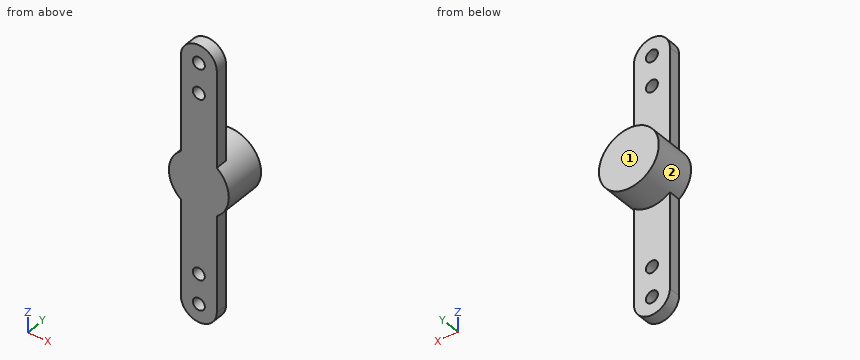
Autodesk Inventor part; units mm, degrees
ref_plane "YZ Plane" through (0, 0, 0) normal (1, 0, 0) x (0, 1, 0)
ref_plane "XZ Plane" through (0, 0, 0) normal (0, 1, 0) x (-1, 0, 0)
ref_plane "XY Plane" through (0, 0, 0) normal (0, 0, 1) x (1, 0, 0)
sketch "スケッチ1" plane through (0, 0, 0) normal (0, 1, 0) x (-1, 0, 0)
  circle A0 centre (0, 0) radius 2.5
  circle A1 centre (0, 10) radius 1.5
  circle A2 centre (0, -10) radius 1.5
  line L0 (1.5, 10) -> (1.5, 2)
  line L1 (-1.5, 10) -> (-1.5, 2)
  line L2 (-1.5, -2) -> (-1.5, -10)
  line L3 (1.5, -2) -> (1.5, -10)
  dimension "d0" = 5
  dimension "d1" = 3
  dimension "d2" = 3
  dimension "d3" = 10
  dimension "d4" = 10
extrude "押し出し1" add sketch "スケッチ1" along normal blind 1
sketch "スケッチ2" plane through (0, 1, 0) normal (0, 1, 0) x (1, 0, 0)
  arc A0 (-1.5, 2) -> (-1.5, -2) centre (0, 0) ccw
  circle A1 centre (0, 0) radius 2.5
extrude "押し出し2" add sketch "スケッチ2" along normal blind 2.5
sketch "スケッチ3" plane through (0, 0, 0) normal (0, -1, 0) x (1, 0, 0)
  arc A0 (1.5, 10) -> (-1.5, 10) centre (0, 10) ccw
  arc A1 (-1.5, -10) -> (1.5, -10) centre (0, -10) ccw
  point P0 (0, 7.5)
  point P1 (0, -7.5)
  dimension "d9" = 2.5
  dimension "d10" = 2.5
hole "穴1" at (0, 0, 10) at (0, 0, -10) at (0, 0, 7.5) at (0, 0, -7.5) direction (0, 1, 0) diameter 1 end through all
properties part number "ナックル"
The listing builds one solid part. Answer for the finished solid, in the listing's coordinates (mm). Face numbers are marked on the shaded views. A direction names the side the tool comes from. Give positions to 0.01 mm unless a question says otherwise; leave off trailing zeros. Write each loop counter-clockwise with the first axis right and the second up, starting at its lowest first coordinate (ties: lowest second). Pieces come first, ordered by that corner, then holes. Notation, with made-up numbers: (76, 5.25) -> (100, 5.25) arc R15 ccw to (100, 20.25) -> close; hole circle Ø8 at (7, 65). An arc over 180 degrees is marked (long way). One line per question, with ' | ' between items. Start each with the question number.
1. Given pin 1 Ø1.5 at (x, z) = (0, -8.5) entering from +Y; pin 2 Ø1 at (x, y) = (-1, 1) entering from +Z; pin 3 Ø1.1 at (y, z) = (0.5, -7) entering from -X; pin 4 Ø1.5 at (x, y) = (0.5, 1.5) entering from +Z, each flat-ended and moving along its own axis, determine where each tip first touches the part or whether it passes through.
2. Section C-C (y = 0.7) is taken. Determine the outline of the cut face in (x, z), plus the area to 3 significant figures.
3. Find the intervals of material crossed by probe 1 along Z at (x, y) = (0, 0.7); probe 2 along X at (y, z) = (0.5, -10); probe 3 along Y at (x, z) = (0.45, -5.5), in increasing order.
4. Section B-B (z = 7.5) is taken. Determine the outline of the cut face in (x, y), plus the area to 3 significant figures.
5. For the marked faces 1 and 2, determine the directions among +Z, -Z, +X, -X, +Y, -Y from which every point of the face is accessible in a straight line to the end or side of a thin tool.
6. Section A-A (x = 0) is taken. Determine the outline of the cut face in (y, z), plus the area to 3 significant figures.
7. Section D-D (x = -1.1) is taken. Determine the outline of the cut face in (y, z) (3 decimals), plus the area to 3 significant figures.
Response values:
1) pin 1: y = 1 | pin 2: z = 11.41 | pin 3: x = -1.5 | pin 4: z = 11.5
2) outline: (-1.5, -10) arc R1.5 ccw to (1.5, -10) -> (1.5, -2) arc R2.5 ccw to (1.5, 2) -> (1.5, 10) arc R1.5 ccw to (-1.5, 10) -> (-1.5, 2) arc R2.5 ccw to (-1.5, -2) -> close; hole circle Ø1 at (0, -10); hole circle Ø1 at (0, -7.5); hole circle Ø1 at (0, 7.5); hole circle Ø1 at (0, 10) | area: 69.5 mm2
3) probe 1: -11.5 to -10.5, -9.5 to -8, -7 to 7, 8 to 9.5, 10.5 to 11.5 | probe 2: -1.5 to -0.5, 0.5 to 1.5 | probe 3: 0 to 1
4) outline: (-1.5, 0) -> (-0.5, 0) -> (-0.5, 1) -> (-1.5, 1) -> close; (0.5, 0) -> (1.5, 0) -> (1.5, 1) -> (0.5, 1) -> close | area: 2.00 mm2
5) face 1: +Z, -Z, +X, -X, +Y | face 2: +Y
6) outline: (0, -11.5) -> (1, -11.5) -> (1, -10.5) -> (0, -10.5) -> close; (0, -9.5) -> (1, -9.5) -> (1, -8) -> (0, -8) -> close; (0, -7) -> (1, -7) -> (1, -2.5) -> (3.5, -2.5) -> (3.5, 2.5) -> (1, 2.5) -> (1, 7) -> (0, 7) -> close; (0, 8) -> (1, 8) -> (1, 9.5) -> (0, 9.5) -> close; (0, 10.5) -> (1, 10.5) -> (1, 11.5) -> (0, 11.5) -> close | area: 31.5 mm2
7) outline: (0, -11.02) -> (1, -11.02) -> (1, -2.245) -> (3.5, -2.245) -> (3.5, 2.245) -> (1, 2.245) -> (1, 11.02) -> (0, 11.02) -> close | area: 33.3 mm2
